Work out the finished part from the listing and answer in its coordinate system (mm). A direction names the side the tool comes from. Round coordinates to 2 decimals unless told otherwise and drop trailing zeros. Write each loop counter-clockwise with the first axis right and the second up, starting at its lowest first coordinate (ties: lowest second). Pieces come first, ordered by that corner, then holes.
from build123d import *

# Parameters (mm, degrees)
SKETCH1_W           = 110.344434204
SKETCH1_H           = 110.344434204
SKETCH1_R           = 1.6
SKETCH1_W_2         = 20.7
SKETCH1_H_2         = 41.4
BOSS_EXTRUDE1_DEPTH = 3
SKETCH3_W           = 10.2
SKETCH3_H           = 3.2
SKETCH3_W_2         = 3.2
SKETCH3_H_2         = 10.2
CUT_EXTRUDE1_DEPTH  = 4


with BuildPart() as part:
    # Sketch1 → Boss-Extrude1 (new body)
    with BuildSketch(Plane(origin=(0, 0, 0), x_dir=(1, 0, 0), z_dir=(0, 1, 0))):
        with Locations((0, 11.670773756)):
            Rectangle(SKETCH1_W, SKETCH1_H)
        with Locations((-5, 34.6)):
            Circle(SKETCH1_R, mode=Mode.SUBTRACT)
        with Locations((5, 34.6)):
            Circle(SKETCH1_R, mode=Mode.SUBTRACT)
        with Locations((5, -13.9)):
            Circle(SKETCH1_R, mode=Mode.SUBTRACT)
        with Locations((-5, -13.9)):
            Circle(SKETCH1_R, mode=Mode.SUBTRACT)
        with Locations((0, 10.35)):
            Rectangle(SKETCH1_W_2, SKETCH1_H_2, mode=Mode.SUBTRACT)
    extrude(amount=BOSS_EXTRUDE1_DEPTH)

    # Sketch3 → Cut-Extrude1 (cut, through all)
    with BuildSketch(Plane(origin=(0, 0, 0), x_dir=(1, 0, 0), z_dir=(0, 1, 0))):
        with Locations((10, 65.342990858)):
            Rectangle(SKETCH3_W, SKETCH3_H)
        Polygon((24.9, 66.942990858), (55.272217102, 66.942990858), (55.272217102, 36.570773756), (52.072217102, 36.570773756), (52.072217102, 63.742990858), (24.9, 63.742990858), align=None)
        with Locations((53.672217102, 21.670773756)):
            Rectangle(SKETCH3_W_2, SKETCH3_H_2)
        Polygon((24.9, -40.401443346), (52.072217102, -40.401443346), (52.072217102, -13.229226244), (55.272217102, -13.229226244), (55.272217102, -43.601443346), (24.9, -43.601443346), align=None)
        with Locations((53.672217102, 1.670773756)):
            Rectangle(SKETCH3_W_2, SKETCH3_H_2)
        Polygon((-52.072217102, -13.229226244), (-55.272217102, -13.229226244), (-55.272217102, -43.601443346), (-24.9, -43.601443346), (-24.9, -40.401443346), (-52.072217102, -40.401443346), align=None)
        with Locations((-53.672217102, 21.670773756)):
            Rectangle(SKETCH3_W_2, SKETCH3_H_2)
        with Locations((-10, 65.342990858)):
            Rectangle(SKETCH3_W, SKETCH3_H)
        Polygon((-55.272217102, 36.570773756), (-52.072217102, 36.570773756), (-52.072217102, 63.742990858), (-24.9, 63.742990858), (-24.9, 66.942990858), (-55.272217102, 66.942990858), align=None)
        with Locations((-53.672217102, 1.670773756)):
            Rectangle(SKETCH3_W_2, SKETCH3_H_2)
        with Locations((-10, -42.001443346)):
            Rectangle(SKETCH3_W, SKETCH3_H)
        with Locations((10, -42.001443346)):
            Rectangle(SKETCH3_W, SKETCH3_H)
    extrude(amount=CUT_EXTRUDE1_DEPTH, mode=Mode.SUBTRACT)


solid = part.part
Q1. A tool of negligible diameter and unlimited length cuts with its end or side. For faces 5 (the face through (-4.9, 1, 42)), 6 (the face through (-39, 1, -63.743)), 7 (the face through (52.072, 1, -50)), 8 (the face through (-38, 1, 40.401)), 9 (the face through (24.9, 1, 42)), from which of +Z, -Z, +X, -X, +Y, -Y can it reach the whole face along a straight path? Write none if from no direction.
Q2. Find section A-A (z = -34.6). Determine the outline of the cut face in (x, y), plus the area to 3 significant figures.
Q3. Find section B-B (x = 1). Determine the outline of the cut face in (y, z).
Q4. The mould has two halves that part along Z. Classify faces 1 (the face through (54, 1, -26.771)), 2 (the face through (-54, 1, -6.771)), 3 (the face through (54, 1, -36.571)), 4 (the face through (-55.172, 1, 8)): +Z half, -Z half, draft (parallel to the pull), parting line (faces both ways), or undercut.
Q5. Given pin 1 (1.5 mm diameter, centred on x = 54.5, y = 2, fed in from -Z); pin 2 (2.5 mm diameter, centred on x = 5, z = -34.6, fed in from -Y); pin 3 (0.9 mm diameter, centred on y = 1.5, z = 41.5, fed in from +X); pin 4 (1.5 mm diameter, centred on x = 44, y = 1.5, fed in from -Z), each flat-ended and moving along its own axis, determine where each tip first touches the part or whether it passes through.
Q6. Find section C-C (z = 6.5). Determine the outline of the cut face in (x, y).
Q7. Find the intervals of material crossed by L1, parallel to X at y = 1.9, z = -34.6; L2, parallel to Z at x = -5, y = 1; L3, parallel to X at y = 0.9, z = 13.9, in increasing order.
Q8. Find section D-D (y = 2.05). Count the separate pieces of the cut face and the enclosed holes in it, plus the area to 3 significant figures.
Report:
1. face 5: +Z, +Y, -Y
1. face 6: -Z, -X, +Y, -Y
1. face 7: -Z, +X, +Y, -Y
1. face 8: +Z, -X, +Y, -Y
1. face 9: +Z, +X, +Y, -Y
2. outline: (-55.17, 0) - (-6.6, 0) - (-6.6, 3) - (-55.17, 3) - close; (-3.4, 0) - (3.4, 0) - (3.4, 3) - (-3.4, 3) - close; (6.6, 0) - (55.17, 0) - (55.17, 3) - (6.6, 3) - close
2. area: 312 mm2
3. outline: (0, -66.84) - (3, -66.84) - (3, -31.05) - (0, -31.05) - close; (0, 10.35) - (3, 10.35) - (3, 43.5) - (0, 43.5) - close
4. face 1: undercut
4. face 2: undercut
4. face 3: -Z half
4. face 4: draft
5. pin 1: stops at z = -36.57
5. pin 2: passes through
5. pin 3: stops at x = 24.9
5. pin 4: stops at z = -63.74
6. outline: (-55.17, 0) - (-10.35, 0) - (-10.35, 3) - (-55.17, 3) - close; (10.35, 0) - (55.17, 0) - (55.17, 3) - (10.35, 3) - close
7. L1: x = -55.17 to -6.6, -3.4 to 3.4, 6.6 to 55.17
7. L2: z = -63.74 to -36.2, -33 to -31.05, 10.35 to 12.3, 15.5 to 40.4
7. L3: x = -52.07 to -6.6, -3.4 to 3.4, 6.6 to 52.07
8. separate pieces: 1
8. enclosed holes: 5
8. area: 10,300 mm2
